Source: three-view drawing plus pictorial views. Frame: mm from the lowest corner of the part. Give positions to 0.01 mm unless a question says otherwise; leave off trailing zeros. Write each loop counter-clockwise with the first axis right and the second up, starting at its lowest first coordinate (ties: lowest second). Pieces come first, ordered by that corner, then holes. Notation, with made-up numbers: (-38, 65) -> (-19, 65) arc R20 cw to (-19, 90) -> close; hole circle Ø5 at (19, 8.25). An arc over 180 degrees is marked (long way). Use a Markdown table: item, result. Add a question column.
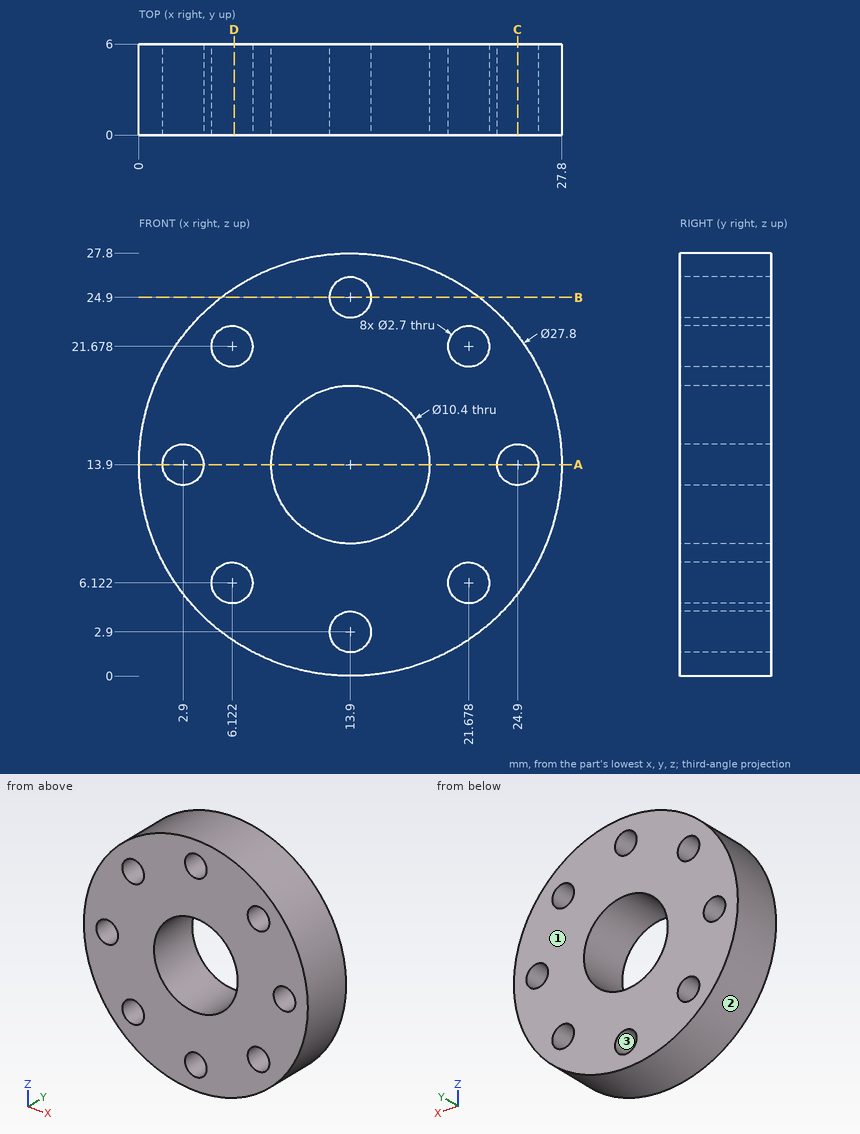
(1) First-contact query: pin 1 Ø1 at (y, z) = (1.5, 8.5) entering from -X. Flat tip, straight axial feed; report the tip coordinate or a pass-through.
(2) Material intervals for L1, parallel to X at y = 3.2, z = 14.75 (1 decimal); L2, parallel to Z at x = 22.75, y = 3.75; L3, parallel to Z at x = 22.5, y = 4.15, sorted ascending.
(3) Cut plane B-B on z = 24.9. Return the cut outline in (x, y), then the cut area to 3 significant figures.
(4) Cut plane D-D on x = 6.25. Return the cut outline in (y, z).
(5) Cut plane A-A on z = 13.9. Return the cut outline in (x, y).
(6) Mould query, pull axis X, two halves, no side actions, for the marked faces 1, 2 and 3. Classes: +X half, -X half, draft (parallel to the pull), parting line (faces both ways), or undercut.
(7) Cut plane C-C on x = 24.9. Return the cut outline in (y, z).
Output:
| question | item | result |
|---|---|---|
| 1 | pin 1 | x = 0.89 |
| 2 | L1 | 0 to 1.9, 3.9 to 8.8, 19 to 23.9, 25.9 to 27.8 |
| 2 | L2 | 3.18 to 5.3, 6.94 to 20.86, 22.5 to 24.62 |
| 2 | L3 | 2.98 to 5.05, 7.19 to 20.61, 22.75 to 24.82 |
| 3 | outline | (5.4, 0) -> (12.55, 0) -> (12.55, 6) -> (5.4, 6) -> close; (15.25, 0) -> (22.4, 0) -> (22.4, 6) -> (15.25, 6) -> close |
| 3 | area | 85.8 mm^2 |
| 4 | outline | (0, 2.29) -> (6, 2.29) -> (6, 4.78) -> (0, 4.78) -> close; (0, 7.47) -> (6, 7.47) -> (6, 20.33) -> (0, 20.33) -> close; (0, 23.02) -> (6, 23.02) -> (6, 25.51) -> (0, 25.51) -> close |
| 5 | outline | (0, 0) -> (1.55, 0) -> (1.55, 6) -> (0, 6) -> close; (4.25, 0) -> (8.7, 0) -> (8.7, 6) -> (4.25, 6) -> close; (19.1, 0) -> (23.55, 0) -> (23.55, 6) -> (19.1, 6) -> close; (26.25, 0) -> (27.8, 0) -> (27.8, 6) -> (26.25, 6) -> close |
| 6 | face 1 | draft |
| 6 | face 2 | parting line |
| 6 | face 3 | undercut |
| 7 | outline | (0, 5.4) -> (6, 5.4) -> (6, 12.55) -> (0, 12.55) -> close; (0, 15.25) -> (6, 15.25) -> (6, 22.4) -> (0, 22.4) -> close |
